Design review of the part built by this model. Coordinates are the model's own, in mm. A direction names the side the tool comes from. Give positions to 0.01 mm unless a question says otherwise; leave off trailing zeros. Order: outer loops, then holes, each group sorted by start corner. A loop starts at its lowest first (then second) coordinate and runs counter-clockwise, first axis right, second up. Notation, with made-up numbers: (60.25, 2.5) -> (97.25, 2.5) arc R26 cw to (97.25, 34.5) -> close; hole circle Ø8 at (10, 66.25). An arc over 180 degrees is marked (long way). One line per item, written item: value. Start each with the question number.
1) Consider section B-B (z = -12.7). State how many separate pieces and enclosed holes the cut face has, plus the area to 3 significant figures.
2) Wall thickness on line 1 along X through (y, z) = (-26.6, -12.7); line 2 along Y through (x, z) = (13, -15) (3 decimals); line 3 along X through (y, z) = (-27, -12): over which ranges is each line inside the solid? List them lowest first. Write a range as from..to.
3) The part is to be moulded in two halves that separate along X. For faces 1 (the face through (-33.834, 4, 1)), 2 (the face through (3.7, 25.4, -15.3)), 3 (the face through (16.97, 0.37, 5.25)), say which applies: released by +X, released by -X, zero draft, split by the parting line, or undercut.
4) Consider section D-D (x = 36.5). State the section outline as (y, z) points (3 decimals).
5) Consider section C-C (z = -19.5). State the section outline as (x, y) points (3 decimals), plus the area to 3 significant figures.
6) For pin 1 (10 mm diameter, centred on x = -24, y = 15, fed in from -Z); pin 2 (2 mm diameter, centred on x = 19, y = -2, fed in from -Z), all flat-tipped, find the tip position at first contact; note any pin that passes through.
7) Tool access review of faces 4 (the face through (0, 15.875, 2)), 5 (the face through (4, -25.4, -10)), 6 (the face through (-18.964, 26.965, -13.182)): name each direction out of +Z, -Z, +X, -X, +Y, -Y from which nothing blocks a thin tool from reaching the whole face with its end or side.
Autodesk Inventor part; units mm, degrees
ref_plane "YZ Plane" through (0, 0, 0) normal (1, 0, 0) x (0, 1, 0)
ref_plane "XZ Plane" through (0, 0, 0) normal (0, 1, 0) x (-1, 0, 0)
ref_plane "XY Plane" through (0, 0, 0) normal (0, 0, 1) x (1, 0, 0)
sketch "Sketch1" plane through (0, 0, 0) normal (0, 0, 1) x (1, 0, 0)
  circle A0 centre (0, 0) radius 15.875
  line L0 (0, 15.875) -> (0, 25.4)
  line L1 (0, 25.4) -> (-33.8337, 25.4)
  line L2 (-33.8337, 25.4) -> (-33.8337, -25.4)
  line L3 (-33.8337, -25.4) -> (0, -25.4)
  line L4 (0, -25.4) -> (0, -15.875)
  line L5 (0, -15.875) -> (0, 15.875)
  line L6 (0, 25.4) -> (42.3663, 25.4)
  line L7 (42.3663, 25.4) -> (42.3663, -25.4)
  line L8 (42.3663, -25.4) -> (0, -25.4)
  line L9 (0, -25.4) -> (0, 25.4)
  line L10 (4.2663, 25.4) -> (4.2663, -25.4) construction
  line L11 (-21.1337, 25.4) -> (-21.1337, -25.4) construction
  line L12 (29.6663, 25.4) -> (29.6663, -25.4) construction
  dimension "d0" = 31.75
  dimension "d1" = 50.8
  dimension "d3" = 4.2663
  dimension "d6" = 38.1
  dimension "d7" = 38.1
  dimension "d8" = 25.4
  dimension "d9" = 25.4
extrude "Extrusion1" add sketch "Sketch1" along normal blind 6.35 contours A0 L0 L6 L7 L8 L4 | A0 L4 L3 L2 L1 L0
chamfer "Chamfer1" distance 6.35 distance2 6.35 1 edges at (-15.875, 0, 0) measured on face at (15.8235, -1.2774, 4.2333)
sketch "Sketch2" plane through (-33.8337, -25.4, 0) normal (-1, 0, 0) x (0, 0, 1)
  line L0 (0, 0) -> (6.35, 0)
  line L1 (6.35, 0) -> (-25.4, 0)
  line L2 (-25.4, 0) -> (-25.4, -3.175)
  line L3 (-25.4, -3.175) -> (6.35, -3.175)
  line L4 (6.35, -3.175) -> (6.35, 0)
  line L5 (6.35, 50.8) -> (-25.4, 50.8)
  line L6 (-25.4, 50.8) -> (-25.4, 53.975)
  line L7 (-25.4, 53.975) -> (6.35, 53.975)
  line L8 (6.35, 53.975) -> (6.35, 50.8)
  line L9 (0, 50.8) -> (0, 0)
  point P0 (0, 25.4)
  dimension "d15" = 3.175
  dimension "d16" = 25.4
extrude "Extrusion2" add sketch "Sketch2" against normal up to surface (76.2 mm away)
sketch "Sketch3" plane through (-33.8337, 28.575, 6.35) normal (0, 1, 0) x (1, 0, 0)
  line L0 (0, 0) -> (0, 31.75)
  line L1 (0, 31.75) -> (76.2, 31.75)
  point P0 (33.8337, 6.35)
  point P1 (12.7, 19.05)
  point P2 (38.1, 19.05)
  point P3 (63.5, 19.05)
  dimension "d19" = 12.7
  dimension "d20" = 25.4
  dimension "d21" = 25.4
  dimension "d22" = 12.7
hole "Hole1" at (-21.1337, 28.575, -12.7) at (4.2663, 28.575, -12.7) at (29.6663, 28.575, -12.7) direction (0, -1, 0) diameter 4.445 end through all
sketch "Sketch4" plane through (0, 0, 0) normal (0, 0, -1) x (-1, 0, 0)
  line L0 (22.225, -15.875) -> (-22.225, -15.875)
  line L1 (-22.225, -15.875) -> (-22.225, 15.875)
  line L2 (-22.225, 15.875) -> (22.225, 15.875)
  line L3 (22.225, 15.875) -> (22.225, -15.875)
  line L4 (22.225, -15.875) -> (-22.225, 15.875) construction
  line L5 (-22.225, -15.875) -> (22.225, 15.875) construction
  circle A0 centre (0, 0) radius 15.875
  circle A1 centre (0, 0) radius 22.225
  point P0 (15.5543, 15.875)
  point P1 (-15.5543, 15.875)
  point P2 (-15.5543, -15.875)
  point P3 (15.5543, -15.875)
extrude "Extrusion3" add sketch "Sketch4" against normal up to surface (6.35 mm away) contours A1 L0 | L2 A1
properties part number "Outer Channel Guide"
Checked values:
1. separate pieces: 8
1. enclosed holes: 0
1. area: 399 mm^2
2. line 1: x = -33.83..-23.36, -18.91..2.04, 6.49..27.44, 31.89..42.37
2. line 2: y = -28.575..-25.4, 25.4..28.575
2. line 3: x = -33.83..-23.24, -19.02..2.16, 6.38..27.56, 31.78..42.37
3. face 1: released by -X
3. face 2: zero draft
3. face 3: undercut
4. outline: (-28.575, -25.4) -> (-25.4, -25.4) -> (-25.4, 0) -> (25.4, 0) -> (25.4, -25.4) -> (28.575, -25.4) -> (28.575, 6.35) -> (-28.575, 6.35) -> close
5. outline: (-33.834, -28.575) -> (42.366, -28.575) -> (42.366, -25.4) -> (-33.834, -25.4) -> close; (-33.834, 25.4) -> (42.366, 25.4) -> (42.366, 28.575) -> (-33.834, 28.575) -> close
5. area: 484 mm^2
6. pin 1: stops at z = 0
6. pin 2: stops at z = 2.12
7. face 4: -Z
7. face 5: -Z, +X, -X
7. face 6: +Y, -Y
